Geometry: see drawing. Coordinates: mm, zero at the bounding-box minimum. A direction names the side the tool comes from. Give positions to 0.01 mm unless a question says otherwise; leave off trailing zeros. Write each loop counter-clockwise with the first axis right and the second up, starting at its lowest first coordinate (ties: lowest second). Pieces come first, ordered by that corner, then holes.
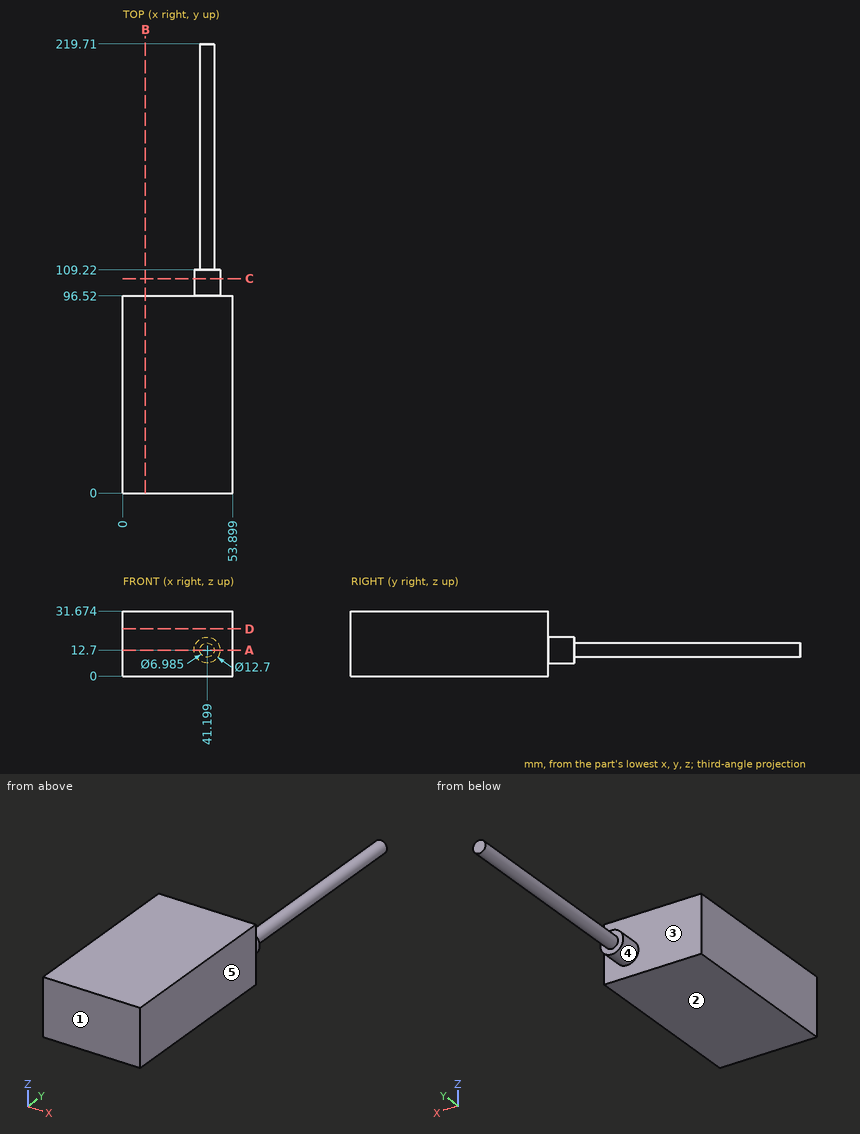
1. Pin query (flat end, axial travel): P1, Ø2, axis at x = 33, y = 92, coming from the -Z side; P2, Ø9.5, axis at x = 16.5, z = 21.5, coming from the +Y side. Return the tip coordinate at first contact, or that it passes through.
2. Line query: probe 1 along Y at (x, z) = (45.5, 30); probe 2 along X at (y, z) = (206, 12.5). Output: solid intervals per line, ascending.
3. Pull-direction query (Y, two-part tool) for the marked faces 1, 2 and 3; classes: pulls with the +Y half, pulls with the -Y half, needs draft (parallel to the pull), parting line crosses it, or undercut.
4. Section query C-C (y = 105). Return loops of the section in (x, z).
5. Access query for the marked faces 4 and 5. Directions: +Z, -Z, +X, -X, +Y, -Y. A direction counts if a zero-diameter tool reaches every point of the face in a straight line with its end or side. Return the directions, or none.
6. Section query D-D (z = 23). Return loops of the section in (x, y), plus the area to 3 significant figures.
7. Section query A-A (z = 12.7). Return loops of the section in (x, y).
8. Section query B-B (x = 11). Return loops of the section in (y, z), plus the area to 3 significant figures.
The answers:
1. P1: stops at z = 0
1. P2: stops at y = 96.52
2. probe 1: y = 0 to 96.52
2. probe 2: x = 37.71 to 44.69
3. face 1: pulls with the -Y half
3. face 2: needs draft
3. face 3: pulls with the +Y half
4. outline: circle Ø12.7 at (41.2, 12.7)
5. face 4: +Y
5. face 5: +Z, -Z, +X, +Y, -Y
6. outline: (0, 0) - (53.9, 0) - (53.9, 96.52) - (0, 96.52) - close
6. area: 5,200 mm2
7. outline: (0, 0) - (53.9, 0) - (53.9, 96.52) - (47.55, 96.52) - (47.55, 109.22) - (44.69, 109.22) - (44.69, 219.71) - (37.71, 219.71) - (37.71, 109.22) - (34.85, 109.22) - (34.85, 96.52) - (0, 96.52) - close
8. outline: (0, 0) - (96.52, 0) - (96.52, 31.67) - (0, 31.67) - close
8. area: 3,060 mm2
